Build history of the part. All positions in model axes, mm. Face numbers are marked on the shaded views. A direction names the side the tool comes from. Give positions to 0.01 mm unless a question says otherwise; leave off trailing zeros. Write each loop counter-clockwise with the first axis right and the second up, starting at its lowest first coordinate (ties: lowest second). Pieces come first, ordered by that corner, then holes. Notation, with made-up numbers: (0.5, 30.5) -> (6.5, 30.5) arc R23 cw to (6.5, 53.5) -> close; hole circle Ø2 at (83.5, 15). An arc over 180 degrees is marked (long way). Put each result on its own line as item: value. Start each with the question number.
Item 1: Tool access for the marked faces 1, 2 and 3: list every direction of +Z, -Z, +X, -X, +Y, -Y with a clear straight run to the whole face (end or side of a thin tool).
Item 2: Drill centre lines: line 1 along Z through (x, y) = (-6, -2.55); line 2 along X through (y, z) = (-0.5, 4); line 3 along Z through (x, y) = (60, 39.5). Where is each one in solid material? Low to high.
Item 3: Slice it at D-D, the plane y = 9. List the corners of the cut face in (x, z).
Item 4: Flat gauge pins, fed straight in: pin 1 Ø2 at (y, z) = (-3, 3.5) entering from +X; pin 2 Ø1 at (x, z) = (58.5, 4.5) entering from -Y; pin 3 Ø12 at (x, z) = (79.5, -3) entering from +Y; pin 4 Ø5 at (x, z) = (6, 8.5) entering from -Y. Where does each tip first touch, or does it go through?
Item 5: Slice it at B-B, the plane x = 60. List the corners of the cut face in (y, z), plus the area to 3 significant figures.
Item 6: Slice it at C-C, the plane y = 44.5. List the corners of the cut face in (x, z).
Item 7: Slice it at A-A, the plane y = 58.16. List the corners of the cut face in (x, z).
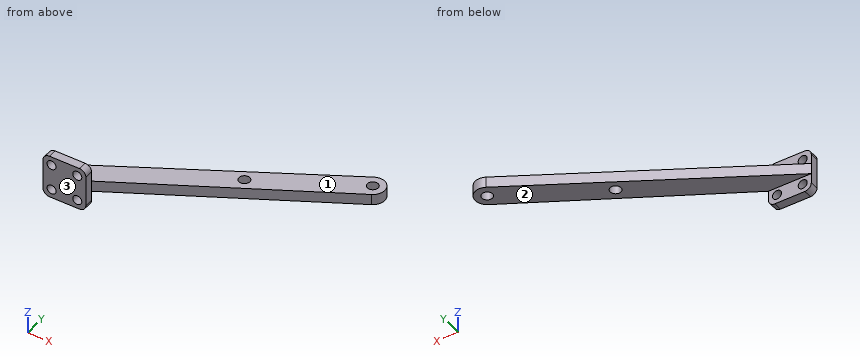
```python
from build123d import *

# Parameters (mm, degrees)
SKETCH1_R           = 2.5
BOSS_EXTRUDE1_DEPTH = 5
SKETCH4_R           = 2.1
BOSS_EXTRUDE3_DEPTH = 4
SKETCH5_R           = 2.5
CUT_EXTRUDE1_DEPTH  = 10


with BuildPart() as part:
    # Sketch1 → Boss-Extrude1 (new body)
    with BuildSketch(Plane.XY):
        with BuildLine():
            Line((10, 0), (-10, 0))
            Line((-10, 0), (99.703266961, 62.930774809))
            ThreePointArc((99.703266961, 62.930774809), (107.223867063, 60.873782586), (105.130769502, 53.363151088))
            Line((105.130769502, 53.363151088), (10, 0))
        make_face()
        with Locations((102.44, 58.16)):
            Circle(SKETCH1_R, mode=Mode.SUBTRACT)
    extrude(amount=BOSS_EXTRUDE1_DEPTH)

    # Sketch4 → Boss-Extrude3 (add)
    with BuildSketch(Plane.XZ):
        with BuildLine():
            Line((7, -7.5), (-7, -7.5))
            ThreePointArc((-7, -7.5), (-9.121320344, -6.621320344), (-10, -4.5))
            Line((-10, -4.5), (-10, 9.5))
            ThreePointArc((-10, 9.5), (-9.121320344, 11.621320344), (-7, 12.5))
            Line((-7, 12.5), (7, 12.5))
            ThreePointArc((7, 12.5), (9.121320344, 11.621320344), (10, 9.5))
            Line((10, 9.5), (10, -4.5))
            ThreePointArc((10, -4.5), (9.121320344, -6.621320344), (7, -7.5))
        make_face()
        with Locations((-6, 8.5)):
            Circle(SKETCH4_R, mode=Mode.SUBTRACT)
        with Locations((5.99988022, 8.5)):
            Circle(SKETCH4_R, mode=Mode.SUBTRACT)
        with Locations(Location((5.99988022, -3.5, 0), (0, 0, 180))):
            Circle(SKETCH4_R, mode=Mode.SUBTRACT)
        with Locations(Location((-6, -3.5, 0), (0, 0, 180))):
            Circle(SKETCH4_R, mode=Mode.SUBTRACT)
    extrude(amount=BOSS_EXTRUDE3_DEPTH)

    # Sketch5 → Cut-Extrude1 (cut)
    with BuildSketch(Plane.XY.offset(5)):
        with Locations((58.832282615, 33.698459075)):
            Circle(SKETCH5_R)
    extrude(amount=-CUT_EXTRUDE1_DEPTH, mode=Mode.SUBTRACT)


solid = part.part
```
Values follow:
1. face 1: +Z, +X, -X, +Y
1. face 2: -Z, +X, -X, +Y
1. face 3: +Z, -Z, +X, -X, -Y
2. line 1: -7.5 to -5.6, -1.4 to 6.4, 10.6 to 12.5
2. line 2: -10 to 10
2. line 3: 0 to 5
3. outline: (5.69, 0) -> (26.04, 0) -> (26.04, 5) -> (5.69, 5) -> close
4. pin 1: x = 10
4. pin 2: y = 26.93
4. pin 3: y = 54.32
4. pin 4: y = -4
5. outline: (28.05, 0) -> (31.49, 0) -> (31.49, 5) -> (28.05, 5) -> close; (35.91, 0) -> (40.16, 0) -> (40.16, 5) -> (35.91, 5) -> close
5. area: 38.4 mm2
6. outline: (67.57, 0) -> (89.33, 0) -> (89.33, 5) -> (67.57, 5) -> close
7. outline: (91.39, 0) -> (99.94, 0) -> (99.94, 5) -> (91.39, 5) -> close; (104.94, 0) -> (107.94, 0) -> (107.94, 5) -> (104.94, 5) -> close
